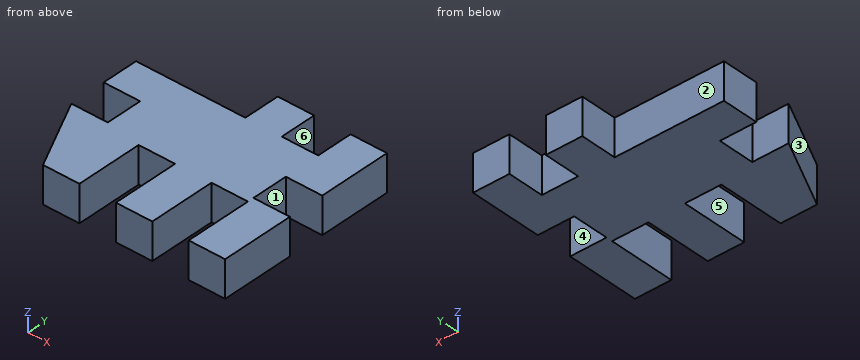
from build123d import *

# Parameters (mm, degrees)
F1_DEPTH = 10


with BuildPart() as f1:
    # F0 (on Top) → F1 (new body)
    with BuildSketch(Plane.XY):
        Polygon((-10, 29.483898), (-29.91453, 29.483898), (-40, 29.483898), (-40, 19.483898), (-30, 19.483898), (-30, 9.483898), (-40, 9.483898), (-30, -10.516102), (-20, -10.516102), (-20, 7.777781), (-10, 7.777781), (-10, -10.516102), (0, -10.516102), (0, 7.777781), (10, 7.777781), (10, -10.516102), (20, -10.516102), (20, 9.483898), (10, 9.483898), (10, 19.483898), (20, 19.483898), (20, 39.483898), (10, 39.483898), (10, 29.483898), (0, 29.483898), (0, 39.483898), (-10, 39.483898), align=None)
    extrude(amount=F1_DEPTH)


solid = f1.part
Check sheet for the modelled part. Datum: model origin and axes. Units: mm. Face numbers are marked on the shaded views. A direction names the side the tool comes from. Round coordinates to 2 decimals unless told otherwise and drop trailing zeros. Loops run counter-clockwise (first coordinate to the right, second up) from the corner with the lowest first, then second, coordinate; pieces in that order, holes last.
1. Sectioned sample at C-C on x = -25. Record the boundary of the cut face in (y, z).
2. Sectioned sample at A-A on y = 36. Record the boundary of the cut face in (x, z).
3. Sectioned sample at D-D on y = 17. Record the boundary of the cut face in (x, z).
4. Sectioned sample at B-B on z = 9.25. Record the boundary of the cut face in (x, y), and give its area (3 significant figures).
5. Mould release check, pull along Y, two halves, no side actions. Record for the marked faces 1, 2 and 3: released by +Y, released by -Y, zero draft, split by the parting line, or undercut.
6. Set-up check for the marked faces 4, 5 and 6: record each of +Z, -Z, +X, -X, +Y, -Y from which the full face is reachable in a straight line by a thin tool's end or side.
7. Gauge pin test, flat ends, axial feed: pin 1 Ø5 at (x, z) = (-16.5, 5) entering from -Y; pin 2 Ø3 at (y, z) = (12.5, 6.5) entering from -X; pin 3 Ø3 at (y, z) = (36.5, 5) entering from -X. Record the tip position at first contact, or that the pin passes through.
8. Scan lines: probe 1 along X at (y, z) = (32.5, 5.75); probe 2 along Y at (x, z) = (13.5, 3.75); probe 3 along X at (y, z) = (11, 4). Record each from-to range of solid material in increasing order.
Recorded:
1. outline: (-10.52, 0) - (29.48, 0) - (29.48, 10) - (-10.52, 10) - close
2. outline: (-10, 0) - (0, 0) - (0, 10) - (-10, 10) - close; (10, 0) - (20, 0) - (20, 10) - (10, 10) - close
3. outline: (-30, 0) - (10, 0) - (10, 10) - (-30, 10) - close
4. outline: (-40, 9.48) - (-30, -10.52) - (-20, -10.52) - (-20, 7.78) - (-10, 7.78) - (-10, -10.52) - (0, -10.52) - (0, 7.78) - (10, 7.78) - (10, -10.52) - (20, -10.52) - (20, 9.48) - (10, 9.48) - (10, 19.48) - (20, 19.48) - (20, 39.48) - (10, 39.48) - (10, 29.48) - (0, 29.48) - (0, 39.48) - (-10, 39.48) - (-10, 29.48) - (-40, 29.48) - (-40, 19.48) - (-30, 19.48) - (-30, 9.48) - close
4. area: 1,930 mm2
5. face 1: undercut
5. face 2: released by +Y
5. face 3: released by -Y
6. face 4: +Z, -Z, +X
6. face 5: +Z, -Z, -Y
6. face 6: +Z, -Z, +Y
7. pin 1: stops at y = 7.78
7. pin 2: stops at x = -30
7. pin 3: stops at x = -10
8. probe 1: x = -10 to 0, 10 to 20
8. probe 2: y = -10.52 to 9.48, 19.48 to 39.48
8. probe 3: x = -30 to 10
